Here's how the part is built. I have some questions about the finished solid (model axes, mm). Face numbers are marked on the shaded views. A direction names the side the tool comes from. Coordinates: 2 decimals unless noted, no trailing zeros. Write each loop counter-clockwise with the first axis right and the second up, starting at its lowest first coordinate (ties: lowest second). Pieces come first, ordered by that corner, then holes. Notation, with made-up numbers: (44, 44) - (57, 44) arc R20 ccw to (57, 64) - close; hole circle Ø10 at (73, -26.75). An arc over 180 degrees is marked (long way). Answer in a Markdown table with one row per item. Add a question column.
Item 1: Imagine slicing it at C-C (x = 8.5). Please give me the cut outline in (y, z).
Item 2: We'd pull the mould along Z, two halves only. Please class the marked faces 4, 5, 6 and 7: +Z half, -Z half, draft (parallel to the pull), parting line (faces both ways), or undercut.
Item 3: Imagine slicing it at B-B (y = 40.5). Please give me the cut outline in (x, z).
Item 4: Imagine slicing it at D-D (z = -14). State how many separate pieces and enclosed holes the cut face has, plus the area to 3 significant figures.
Item 5: I'm going to push flat-ended pins straight in: pin 1 (7 mm diameter, centred on x = 0, z = -6, fed in from +Y); pin 2 (3.5 mm diameter, centred on y = 0.06, z = -18.9, fed in from +X); pin 3 (3 mm diameter, centred on x = 17, z = -5, fed in from -Y). Where does each tip first touch, or does it pass through?
Item 6: Imagine slicing it at A-A (x = 19.5). Please give me the cut outline in (y, z).
Item 7: If I drill on probe 1 along X at (y, z) = (3.25, -6); probe 2 along Z at (x, y) = (-22.75, 0.06) (3 decimals); probe 3 along Y at (x, z) = (-23.5, -9.5), over which ranges is the centre line in solid material (lowest first)? Write a range as from..to.
Item 8: Which directions (+Z, -Z, +X, -X, +Y, -Y) give clear straight access to the entire face, cutting with the end or side of a thin tool? Please do the marked faces 1, 2 and 3.
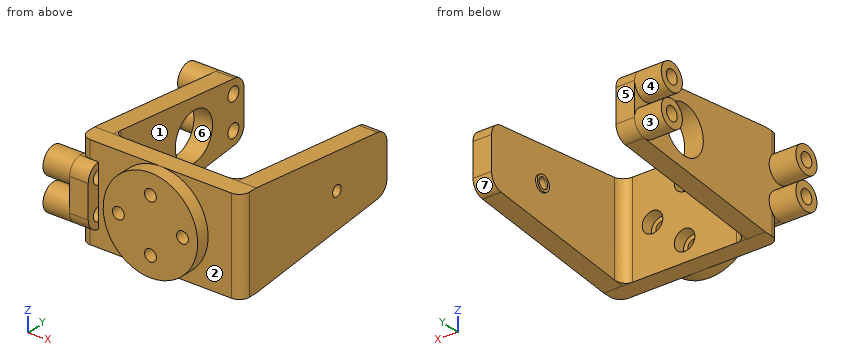
from build123d import *

# Parameters (mm, degrees)
GIMBAL_MOUNT_BODY_DEPTH        = 28
SKETCH7_R                      = 7.05
SERVO_GEAR_MOUND_CUT_OUT_DEPTH = 5.5
BOSS_EXTRUDE6_DEPTH            = 5.5
BOSS_EXTRUDE7_START            = 7.9
SKETCH15_R                     = 4
BOSS_EXTRUDE7_DEPTH            = 7.9
SKETCH17_R                     = 1.6
CUT_EXTRUDE2_DEPTH             = 5.5
SKETCH19_R                     = 14
BOSS_EXTRUDE9_DEPTH            = 3.94
SKETCH20_R                     = 1.75
CUT_EXTRUDE4_DEPTH             = 9.44
SKETCH21_R                     = 2.055
CUT_EXTRUDE5_DEPTH             = 13.4
SKETCH30_R                     = 2.3
SKETCH30_R_2                   = 1.6
BOSS_EXTRUDE10_DEPTH           = 0.5
CUT_EXTRUDE11_DEPTH            = 82.696849282
SKETCH29_R                     = 3.05
CUT_EXTRUDE12_DEPTH            = 3.5
CUT_EXTRUDE7_DEPTH             = 82.696849282
FILLET4_R                      = 3
FILLET5_R                      = 4


# Some blends are built 0.0001 mm under size
with BuildPart() as part:
    # Sketch6 → Gimbal Mount Body (new body)
    with BuildSketch(Plane.XY):
        Polygon((0, 0), (-14, 0), (-23.928932188, 0), (-23.928932188, 9.928932188), (-23.928932188, 60), (-18.428932188, 60), (-18.428932188, 12), (-18.428932188, 5.5), (-11.928932188, 5.5), (0, 5.5), align=None)
    gimbal_mount_body = extrude(amount=-GIMBAL_MOUNT_BODY_DEPTH)

    # Gimbal Mount Body Mirror: Gimbal Mount Body across plane
    add(gimbal_mount_body.mirror(Plane(origin=(0, 0, 0), x_dir=(0, 0, 1), z_dir=(1, 0, 0))))

    # Sketch7 → Servo Gear Mound Cut Out (cut)
    with BuildSketch(Plane.ZY.offset(23.928932188)):
        with Locations(Location((-14, 36, 0), (0, 0, 270))):
            Circle(SKETCH7_R)
    extrude(amount=-SERVO_GEAR_MOUND_CUT_OUT_DEPTH, mode=Mode.SUBTRACT)

    # Sketch14 → Boss-Extrude6 (add)
    with BuildSketch(Plane.ZY.offset(23.928932188)):
        with BuildLine():
            Line((-18.9, -3.94), (-9.1, -3.94))
            ThreePointArc((-9.1, -3.94), (-6.29286623, -2.78956137), (-5.100450025, 0))
            Line((-5.100450025, 0), (-22.899549975, 0))
            ThreePointArc((-22.899549975, 0), (-21.70713377, -2.78956137), (-18.9, -3.94))
        make_face()
    extrude(amount=-BOSS_EXTRUDE6_DEPTH)

    # Sketch15 → Boss-Extrude7 (add)
    with BuildSketch(Plane.ZY.offset(23.928932188).offset(BOSS_EXTRUDE7_START)):
        with Locations((-18.9, 50.94)):
            Circle(SKETCH15_R)
        with Locations((-9.1, 50.94)):
            Circle(SKETCH15_R)
        with Locations((-18.9, 0.06)):
            Circle(SKETCH15_R)
        with Locations((-9.1, 0.06)):
            Circle(SKETCH15_R)
    extrude(amount=-BOSS_EXTRUDE7_DEPTH)

    # Sketch17 → Cut-Extrude2 (cut)
    with BuildSketch(Plane(origin=(23.928932188, 0, 0), x_dir=(0, 0, -1), z_dir=(1, 0, 0))):
        with Locations((14, 36)):
            Circle(SKETCH17_R)
    extrude(amount=-CUT_EXTRUDE2_DEPTH, mode=Mode.SUBTRACT)

    # Sketch19 → Boss-Extrude9 (add)
    with BuildSketch(Plane.XZ):
        with Locations(Location((0, -14, 0), (0, 0, 270))):
            Circle(SKETCH19_R)
    extrude(amount=BOSS_EXTRUDE9_DEPTH)

    # Sketch20 → Cut-Extrude4 (cut)
    with BuildSketch(Plane.XZ.offset(3.94)):
        with Locations(Location((0, -6, 0), (0, 0, 270))):
            Circle(SKETCH20_R)
        with Locations(Location((-9.5, -14, 0), (0, 0, 270))):
            Circle(SKETCH20_R)
        with Locations(Location((9.5, -14, 0), (0, 0, 270))):
            Circle(SKETCH20_R)
        with Locations(Location((0, -22, 0), (0, 0, 270))):
            Circle(SKETCH20_R)
    extrude(amount=-CUT_EXTRUDE4_DEPTH, mode=Mode.SUBTRACT)

    # Sketch21 → Cut-Extrude5 (cut)
    with BuildSketch(Plane.ZY.offset(31.828932188)):
        with Locations((-18.9, 50.94)):
            Circle(SKETCH21_R)
        with Locations((-9.1, 50.94)):
            Circle(SKETCH21_R)
        with Locations((-9.1, 0.06)):
            Circle(SKETCH21_R)
        with Locations((-18.9, 0.06)):
            Circle(SKETCH21_R)
    extrude(amount=-CUT_EXTRUDE5_DEPTH, mode=Mode.SUBTRACT)

    # Sketch30 → Boss-Extrude10 (add)
    with BuildSketch(Plane.ZY.offset(-18.428932188)):
        with Locations(Location((-14, 36, 0), (0, 0, 180))):
            Circle(SKETCH30_R)
        with Locations(Location((-14, 36, 0), (0, 0, 180))):
            Circle(SKETCH30_R_2, mode=Mode.SUBTRACT)
    extrude(amount=BOSS_EXTRUDE10_DEPTH)

    # Sketch28 → Cut-Extrude11 (cut, through all)
    with BuildSketch(Plane.ZY.offset(23.928932188)):
        Polygon((0, 5.5), (-6.087027099, 60), (0, 60), align=None)
        Polygon((-28, 5.5), (-21.912972901, 60), (-28, 60), align=None)
    extrude(amount=-CUT_EXTRUDE11_DEPTH, mode=Mode.SUBTRACT)

    # Sketch29 → Cut-Extrude12 (cut)
    with BuildSketch(Plane(origin=(0, 5.5, 0), x_dir=(1, 0, 0), z_dir=(0, 1, 0))):
        with Locations(Location((0, 22, 0), (0, 0, 270))):
            Circle(SKETCH29_R)
        with Locations(Location((-9.5, 14, 0), (0, 0, 270))):
            Circle(SKETCH29_R)
        with Locations(Location((0, 6, 0), (0, 0, 270))):
            Circle(SKETCH29_R)
        with Locations(Location((9.5, 14, 0), (0, 0, 270))):
            Circle(SKETCH29_R)
    extrude(amount=-CUT_EXTRUDE12_DEPTH, mode=Mode.SUBTRACT)

    # Sketch23 → Cut-Extrude7 (cut, through all)
    with BuildSketch(Plane.ZY.offset(23.928932188)):
        Polygon((-21.912972901, 60), (-6.087027099, 60), (-5.521882932, 54.94), (-22.478117068, 54.94), align=None)
    extrude(amount=-CUT_EXTRUDE7_DEPTH, mode=Mode.SUBTRACT)

    # Fillet4
    # the kernel refuses this fillet: 3 mm, written as the material it adds along each edge
    with BuildSketch(Plane(origin=(-18.428932188, 5.5, 0), x_dir=(1, 0, 0), z_dir=(0, 0, -1))) as fillet4_piece_1_section:
        with BuildLine():
            CenterArc((FILLET4_R, -FILLET4_R), FILLET4_R, 90, 90)
            Line((0, -FILLET4_R), (-FILLET4_R * 0.02, -FILLET4_R))
            Line((-FILLET4_R * 0.02, -FILLET4_R), (-FILLET4_R * 0.02, FILLET4_R * 0.02))
            Line((-FILLET4_R * 0.02, FILLET4_R * 0.02), (FILLET4_R, FILLET4_R * 0.02))
            Line((FILLET4_R, FILLET4_R * 0.02), (FILLET4_R, 0))
        make_face()
    fillet4_piece_1 = extrude(amount=28, mode=Mode.PRIVATE)
    fillet4_piece_1 = split(fillet4_piece_1, bisect_by=Plane(origin=(-17.747779905, 7.711892033, -27.75295694), z_dir=(0, -0.11099840059468292, 0.9938205849475158)), keep=Keep.TOP, mode=Mode.PRIVATE)
    fillet4_piece_1 = split(fillet4_piece_1, bisect_by=Plane(origin=(-17.747779905, 7.711892033, -0.24704306), z_dir=(0, -0.11099840059468276, -0.9938205849475158)), keep=Keep.TOP, mode=Mode.PRIVATE)
    add(fillet4_piece_1)
    with BuildSketch(Plane(origin=(18.428932188, 5.5, 0), x_dir=(-1, 0, 0), z_dir=(0, 0, -1))) as fillet4_piece_2_section:
        with BuildLine():
            CenterArc((FILLET4_R, FILLET4_R), FILLET4_R, 180, 90)
            Line((0, FILLET4_R), (-FILLET4_R * 0.02, FILLET4_R))
            Line((-FILLET4_R * 0.02, FILLET4_R), (-FILLET4_R * 0.02, -FILLET4_R * 0.02))
            Line((-FILLET4_R * 0.02, -FILLET4_R * 0.02), (FILLET4_R, -FILLET4_R * 0.02))
            Line((FILLET4_R, -FILLET4_R * 0.02), (FILLET4_R, 0))
        make_face()
    fillet4_piece_2 = extrude(amount=28, mode=Mode.PRIVATE)
    fillet4_piece_2 = split(fillet4_piece_2, bisect_by=Plane(origin=(17.747779905, 7.711892033, -27.75295694), z_dir=(0, -0.11099840059468292, 0.9938205849475158)), keep=Keep.TOP, mode=Mode.PRIVATE)
    fillet4_piece_2 = split(fillet4_piece_2, bisect_by=Plane(origin=(17.747779905, 7.711892033, -0.24704306), z_dir=(0, -0.11099840059468276, -0.9938205849475158)), keep=Keep.TOP, mode=Mode.PRIVATE)
    add(fillet4_piece_2)
    # the kernel refuses this fillet: 3 mm, written as the material it takes off along each edge
    with BuildSketch(Plane(origin=(-23.928932188, 0, -19.899549975), x_dir=(1, 0, 0), z_dir=(0, 0, -1))) as fillet4_2_piece_1_section:
        with BuildLine():
            CenterArc((FILLET4_R, -FILLET4_R), FILLET4_R, 90, 90)
            Line((0, -FILLET4_R), (-FILLET4_R * 0.02, -FILLET4_R))
            Line((-FILLET4_R * 0.02, -FILLET4_R), (-FILLET4_R * 0.02, FILLET4_R * 0.02))
            Line((-FILLET4_R * 0.02, FILLET4_R * 0.02), (FILLET4_R, FILLET4_R * 0.02))
            Line((FILLET4_R, FILLET4_R * 0.02), (FILLET4_R, 0))
        make_face()
    fillet4_2_piece_1 = extrude(amount=11.100450025, mode=Mode.PRIVATE)
    fillet4_2_piece_1 = fillet4_2_piece_1 - Plane(origin=(-23.256393846, 0.06, -18.9), x_dir=(0, -0.014999999999998508, -0.999887493671163), z_dir=(-1, 0, 0)) * Cylinder(4, 35, mode=Mode.PRIVATE)
    add(fillet4_2_piece_1, mode=Mode.SUBTRACT)
    with BuildSketch(Plane(origin=(23.928932188, 0, 3), x_dir=(0, 1, 0), z_dir=(0, 0, -1))) as fillet4_2_piece_2:
        with BuildLine():
            CenterArc((FILLET4_R, -FILLET4_R), FILLET4_R, 90, 90)
            Line((0, -FILLET4_R), (-FILLET4_R * 0.02, -FILLET4_R))
            Line((-FILLET4_R * 0.02, -FILLET4_R), (-FILLET4_R * 0.02, FILLET4_R * 0.02))
            Line((-FILLET4_R * 0.02, FILLET4_R * 0.02), (FILLET4_R, FILLET4_R * 0.02))
            Line((FILLET4_R, FILLET4_R * 0.02), (FILLET4_R, 0))
        make_face()
    extrude(amount=34, mode=Mode.SUBTRACT)
    with BuildSketch(Plane(origin=(-23.928932188, 0, 3), x_dir=(1, 0, 0), z_dir=(0, 0, -1))) as fillet4_2_piece_3_section:
        with BuildLine():
            CenterArc((FILLET4_R, -FILLET4_R), FILLET4_R, 90, 90)
            Line((0, -FILLET4_R), (-FILLET4_R * 0.02, -FILLET4_R))
            Line((-FILLET4_R * 0.02, -FILLET4_R), (-FILLET4_R * 0.02, FILLET4_R * 0.02))
            Line((-FILLET4_R * 0.02, FILLET4_R * 0.02), (FILLET4_R, FILLET4_R * 0.02))
            Line((FILLET4_R, FILLET4_R * 0.02), (FILLET4_R, 0))
        make_face()
    fillet4_2_piece_3 = extrude(amount=11.100450025, mode=Mode.PRIVATE)
    fillet4_2_piece_3 = fillet4_2_piece_3 - Plane(origin=(-23.256393341, 0.06, -9.1), x_dir=(0, -1, 0), z_dir=(-1, 0, 0)) * Cylinder(4, 35, mode=Mode.PRIVATE)
    add(fillet4_2_piece_3, mode=Mode.SUBTRACT)

    # Fillet5
    fillet5_edges = [part.edges().sort_by_distance(p)[0] for p in [
        (21.178932188, 54.94, -5.521882932),
        (21.178932188, 54.94, -22.478117068),
        (-21.178932188, 54.94, -22.478117068),
        (-21.178932188, 54.94, -5.521882932),
    ]]
    fillet(fillet5_edges, radius=FILLET5_R - 0.0001)  # a hair under: the kernel refuses the full size


solid = part.part
Here are the results:
| question | item | result |
|---|---|---|
| 1 | outline | (-3.94, -25.12) - (0, -25.12) - (0, -28) - (5.5, -28) - (5.5, -16.88) - (2, -16.88) - (2, -15.44) - (-3.94, -15.44) - close; (-3.94, -12.56) - (2, -12.56) - (2, -11.12) - (5.5, -11.12) - (5.5, 0) - (0, 0) - (0, -2.88) - (-3.94, -2.88) - close |
| 2 | face 4 | undercut |
| 2 | face 5 | draft |
| 2 | face 6 | undercut |
| 2 | face 7 | -Z half |
| 3 | outline | (-23.93, -24.09) - (-18.43, -24.09) - (-18.43, -19.43) - (-23.93, -19.43) - close; (-23.93, -8.57) - (-18.43, -8.57) - (-18.43, -3.91) - (-23.93, -3.91) - close; (18.43, -24.09) - (23.93, -24.09) - (23.93, -3.91) - (18.43, -3.91) - close |
| 4 | separate pieces | 5 |
| 4 | enclosed holes | 0 |
| 4 | area | 762 mm2 |
| 5 | pin 1 | stops at y = 5.5 |
| 5 | pin 2 | stops at x = 23.68 |
| 5 | pin 3 | stops at y = 0 |
| 6 | outline | (0, -28) - (5.5, -28) - (51.38, -22.88) arc R4 ccw to (54.94, -18.9) - (54.94, -9.1) arc R4 ccw to (51.38, -5.12) - (5.5, 0) - (0, 0) - close; hole circle Ø3.2 at (36, -14) |
| 7 | probe 1 | x = -23.93..-3.05, 3.05..23.93 |
| 7 | probe 2 | z = -22.9..-20.955, -16.845..-11.155, -7.045..-5.1 |
| 7 | probe 3 | y = -3.94..-1.96, 2.08..30.57, 41.43..48.92, 52.96..54.94 |
| 8 | face 1 | +Z, -Z, +Y |
| 8 | face 2 | +X, -Y |
| 8 | face 3 | -X |
